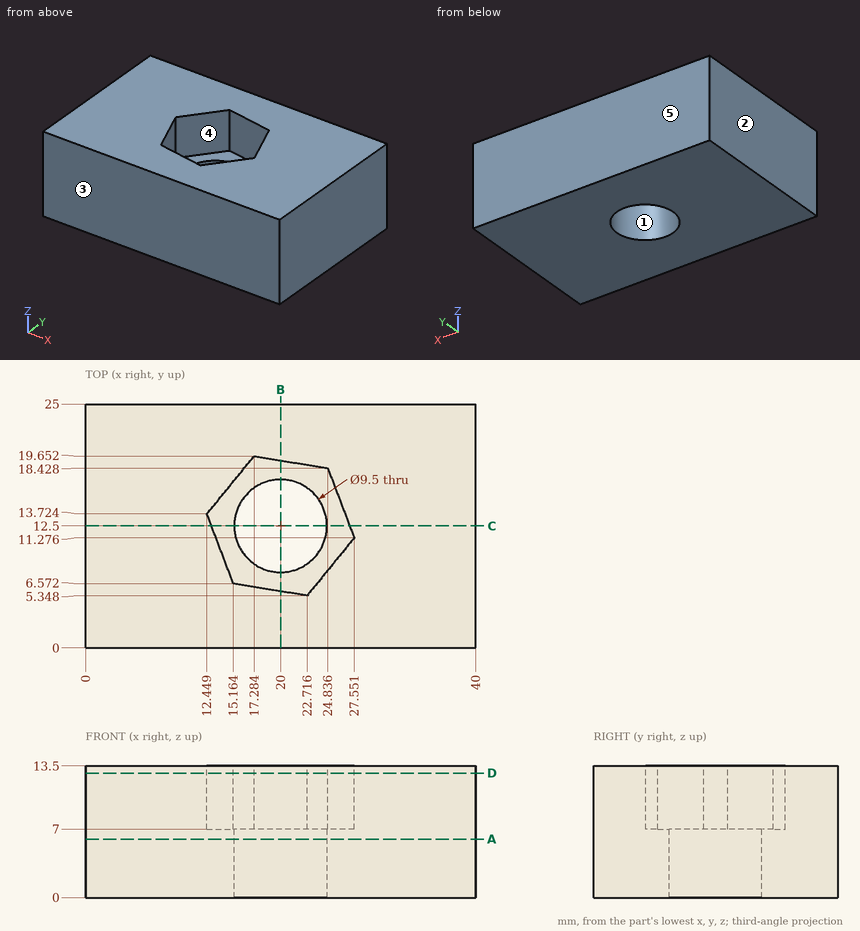
Verification items for this drawing (mm, ordinates from the low corner). A direction names the side the tool comes from. Round coordinates to 2 decimals unless told otherwise and drop trailing zeros. Loops run counter-clockwise (first coordinate to the right, second up) from the corner with the lowest first, then second, coordinate; pieces in that order, holes last. Notation, with made-up numbers: M 67,49 L 117,49 A15 ccw 117,75 Z; hole C -17.5,-13.75 d3. An arc over 180 degrees is marked long. Answer as a JSON object with one key per item and string values.
1. Gauge pin test, flat end, axial feed: P1, Ø7.5, axis at x = 20, y = 12.5, coming from the -Z side. Record the tip position at first contact, or that the pin passes through.
Reply:
{"P1": "passes through"}
2. Scan lines: line 1 (Y direction, x = 20, z = 2.5); line 2 (X direction, y = 8, z = 9.5); line 3 (X direction, y = 16.5, z = 1.25) (1 decimal). Record each from-to range of solid material in increasing order.
Reply:
{"line 1": "y = 0 to 7.75, 17.25 to 25", "line 2": "x = 0 to 14.62, 24.88 to 40", "line 3": "x = 0 to 17.4, 22.6 to 40"}
3. Section check C-C (y = 12.5). Record the boundary of the cut face in (x, z), plus the area to 3 significant figures.
Reply:
{"outline": "M 0,0 L 15.25,0 L 15.25,7 L 12.91,7 L 12.91,13.5 L 0,13.5 Z; M 24.75,0 L 40,0 L 40,13.5 L 27.09,13.5 L 27.09,7 L 24.75,7 Z", "area": "381 mm²"}
4. Section check B-B (x = 20). Record the boundary of the cut face in (y, z).
Reply:
{"outline": "M 0,0 L 7.75,0 L 7.75,7 L 5.79,7 L 5.79,13.5 L 0,13.5 Z; M 17.25,0 L 25,0 L 25,13.5 L 19.21,13.5 L 19.21,7 L 17.25,7 Z"}
5. Mould release check, pull along X, two halves, no side actions. Record for the marked faces 1, 2 and 3: pulls with the +X half, pulls with the -X half, needs draft (parallel to the pull), parting line crosses it, or undercut.
Reply:
{"face 1": "undercut", "face 2": "pulls with the -X half", "face 3": "needs draft"}
6. Section check A-A (z = 6). Record the boundary of the cut face in (x, y).
Reply:
{"outline": "M 0,0 L 40,0 L 40,25 L 0,25 Z; hole C 20,12.5 d9.5"}
7. Access from +Z, -Z, +X, -X, +Y, -Y to the whole of each face (thin tool, end or side, straight path). Record for the marked faces 4 and 5.
Reply:
{"face 4": "+Z", "face 5": "+Z, -Z, +X, -X, +Y"}
8. Section check D-D (z = 12.75). Record the boundary of the cut face in (x, y) (1 decimal), plus the area to 3 significant figures.
Reply:
{"outline": "M 0,0 L 40,0 L 40,25 L 0,25 Z; hole M 12.4,13.7 L 15.2,6.6 L 22.7,5.3 L 27.6,11.3 L 24.8,18.4 L 17.3,19.7 Z", "area": "848 mm²"}
